Geometry check sheet. Reference: the model listing, model coordinates, mm. Face numbers are marked on the shaded views. A direction names the side the tool comes from. Give positions to 0.01 mm unless a question says otherwise; leave off trailing zeros. Loops run counter-clockwise (first coordinate to the right, second up) from the corner with the lowest first, then second, coordinate; pieces in that order, holes last. Notation, with made-up numbers: (-25.75, 21.25) -> (18.25, 21.25) arc R17 cw to (18.25, 34.25) -> close; hole circle Ø1 at (64.25, 45). An arc over 180 degrees is marked (long way). Answer as a JSON object with one key per item and string values.
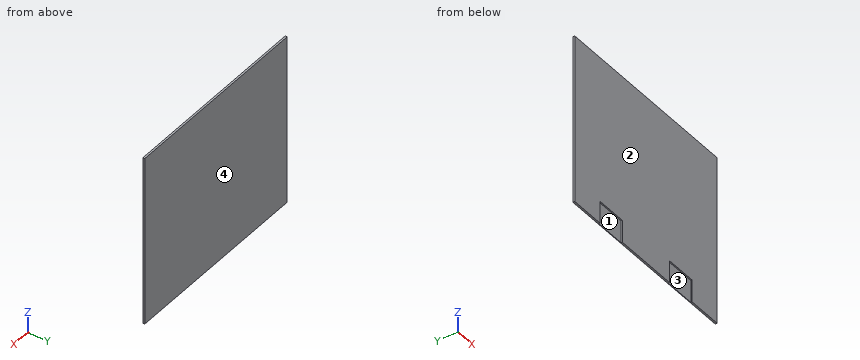
from build123d import *

# Parameters (mm, degrees)
SKETCH1_W           = 315
SKETCH1_H           = 266
BOSS_EXTRUDE1_DEPTH = 3
SKETCH2_W           = 50
SKETCH2_H           = 35
CUT_EXTRUDE1_DEPTH  = 2


with BuildPart() as part:
    # Sketch1 → Boss-Extrude1 (new body)
    with BuildSketch(Plane(origin=(0, 0, 0), x_dir=(1, 0, 0), z_dir=(0, 1, 0))):
        Rectangle(SKETCH1_W, SKETCH1_H)
    extrude(amount=BOSS_EXTRUDE1_DEPTH)

    # Sketch2 → Cut-Extrude1 (cut)
    with BuildSketch(Plane.XZ):
        with Locations((-77.25, -115.5)):
            Rectangle(SKETCH2_W, SKETCH2_H)
    cut_extrude1 = extrude(amount=-CUT_EXTRUDE1_DEPTH, mode=Mode.SUBTRACT)

    # Mirror1: Cut-Extrude1 across plane
    add(cut_extrude1.mirror(Plane(origin=(0, 0, 0), x_dir=(0, 0, 1), z_dir=(1, 0, 0))), mode=Mode.SUBTRACT)


solid = part.part
1) Material ranges on line 1 along Z through (x, y) = (-68.5, 0.55), recorded low to high. Write a range as from..to.
Geometry check:
{"line 1": "z = -98..133"}
2) Draft check along X on the marked faces 3 and 4. Enter one of: pulls with the +X half, pulls with the -X half, needs draft (parallel to the pull), parting line crosses it, or undercut.
Geometry check:
{"face 3": "undercut", "face 4": "needs draft"}
3) Section check C-C on y = 1.3. Record the cut outline in (x, z).
Geometry check:
{"outline": "(-157.5, -133) -> (-102.25, -133) -> (-102.25, -98) -> (-52.25, -98) -> (-52.25, -133) -> (52.25, -133) -> (52.25, -98) -> (102.25, -98) -> (102.25, -133) -> (157.5, -133) -> (157.5, 133) -> (-157.5, 133) -> close"}
4) Section check B-B on x = 85. Record the cut outline in (y, z).
Geometry check:
{"outline": "(0, -98) -> (2, -98) -> (2, -133) -> (3, -133) -> (3, 133) -> (0, 133) -> close"}
5) Tool access check on the marked faces 1 and 2. Record the directions out of +Z, -Z, +X, -X, +Y, -Y that give a thin tool (end or side, any length) a straight path to the whole face; none if there is none.
Geometry check:
{"face 1": "-Z, -Y", "face 2": "+Z, -Z, +X, -X, -Y"}
6) Section check A-A on z = -112.5. Record the cut outline in (x, y), plus the area to 3 significant figures.
Geometry check:
{"outline": "(-157.5, 0) -> (-102.25, 0) -> (-102.25, 2) -> (-52.25, 2) -> (-52.25, 0) -> (52.25, 0) -> (52.25, 2) -> (102.25, 2) -> (102.25, 0) -> (157.5, 0) -> (157.5, 3) -> (-157.5, 3) -> close", "area": "745 mm2"}
7) Depth check by flat-ended pin: P1, Ø10, axis at x = -45, z = -99, coming from the -Y side; P2, Ø0.6, axis at x = -78.5, y = 1, coming from the -Z side. Enter the tip coordinate at first touch or a pass-through.
Geometry check:
{"P1": "stops at y = 0", "P2": "stops at z = -98"}
